```python
from build123d import *

# Parameters (mm, degrees)
F0_R     = 1.5875
F0_R_2   = 3.175
F1_DEPTH = 3.175


with BuildPart() as f1:
    # F0 (on Right) → F1 (new body)
    with BuildSketch(Plane.YZ):
        with BuildLine():
            ThreePointArc((0, 3.175), (2.245064, 2.245064), (3.175, 0))
            ThreePointArc((3.175, 0), (2.245064, -2.245064), (0, -3.175))
            Line((0, -3.175), (18.797582, -6.265861))
            ThreePointArc((18.797582, -6.265861), (13.477869, 0), (18.797582, 6.265861))
            Line((18.797582, 6.265861), (0, 3.175))
        make_face()
        with BuildLine():
            ThreePointArc((0, -3.175), (2.245064, -2.245064), (3.175, 0))
            ThreePointArc((3.175, 0), (2.245064, 2.245064), (0, 3.175))
            ThreePointArc((0, 3.175), (-3.175, 0), (0, -3.175))
        make_face()
        Circle(F0_R, mode=Mode.SUBTRACT)
        with BuildLine():
            ThreePointArc((26.177869, 0), (23.937624, 4.840704), (18.797582, 6.265861))
            ThreePointArc((18.797582, 6.265861), (13.477869, 0), (18.797582, -6.265861))
            ThreePointArc((18.797582, -6.265861), (23.937624, -4.840704), (26.177869, 0))
        make_face()
        with Locations((19.827869, 0)):
            Circle(F0_R_2, mode=Mode.SUBTRACT)
    extrude(amount=F1_DEPTH)


solid = f1.part
```
Source: CAD feature listing. Evaluate the final solid. Frame: model axes, mm. Give positions to 0.01 mm unless a question says otherwise; leave off trailing zeros. Write each loop counter-clockwise with the first axis right and the second up, starting at its lowest first coordinate (ties: lowest second). Pieces come first, ordered by that corner, then holes.
1. Section query B-B (z = -2). Return the cut outline in (x, y) (3 decimals).
2. Section query A-A (x = 1.8). Count the separate pieces of the cut face and the enclosed holes in it, then the cut area to 3 significant figures.
3. First-contact query: pin 1 (1 mm diameter, centred on x = 1.5, y = 4, fed in from -Z); pin 2 (2.5 mm diameter, centred on y = 0, z = 0, fed in from +X). Flat tips, straight axial feed; report the tip coordinate or a pass-through.
4. Section query C-C (y = 18). Return the cut outline in (x, z) (3 decimals), then the cut area to 3 significant figures.
5. Section query D-D (z = 1.25). Return the cut outline in (x, y) (3 decimals), then the cut area to 3 significant figures.
6. Pull-direction query (Y, two-part tool) for faces 1 (the face through (0, 11, 0)), 2 (the face through (1.565, 16.656, 0.14)), 3 (the face through (1.57, -0.34, -1.55)), 4 (the face through (1.57, 9.27, -4.7)); classes: +Y half, -Y half, draft (parallel to the pull), parting line (faces both ways), or undercut.
7. Material intervals for line 1 along Y through (x, z) = (2.9, 1.25); line 2 along Z through (x, y) = (2.8, 22.75); line 3 along Z through (x, y) = (0.65, 22.25), sorted ascending.
Output values:
1. outline: (0, -2.466) - (3.175, -2.466) - (3.175, 17.362) - (0, 17.362) - close; (0, 22.294) - (3.175, 22.294) - (3.175, 25.855) - (0, 25.855) - close
2. separate pieces: 1
2. enclosed holes: 2
2. area: 230 mm2
3. pin 1: stops at z = -3.91
3. pin 2: passes through
4. outline: (0, -6.135) - (3.175, -6.135) - (3.175, -2.596) - (0, -2.596) - close; (0, 2.596) - (3.175, 2.596) - (3.175, 6.135) - (0, 6.135) - close
4. area: 22.5 mm2
5. outline: (0, -2.919) - (3.175, -2.919) - (3.175, -0.979) - (0, -0.979) - close; (0, 0.979) - (3.175, 0.979) - (3.175, 16.909) - (0, 16.909) - close; (0, 22.746) - (3.175, 22.746) - (3.175, 26.054) - (0, 26.054) - close
5. area: 67.2 mm2
6. face 1: draft
6. face 2: undercut
6. face 3: undercut
6. face 4: -Y half
7. line 1: y = -2.92 to -0.98, 0.98 to 16.91, 22.75 to 26.05
7. line 2: z = -5.64 to -1.24, 1.24 to 5.64
7. line 3: z = -5.87 to -2.05, 2.05 to 5.87
